from build123d import *

# Parameters (mm, degrees)
F1_DEPTH = 70
F2_R     = 14.3018330781
F3_DEPTH = 87.7
F4_W     = 40
F4_H     = 30
F5_DEPTH = 60
F7_R     = 5
F8_DEPTH = 86.3


with BuildPart() as f1:
    # F0 (on Right) → F1 (new body, symmetric)
    with BuildSketch(Plane.YZ):
        Polygon((0, 30), (0, 0), (-60, 0), (-60, -30), (10, -30), (10, 30), align=None)
    extrude(amount=F1_DEPTH, both=True)

    # F2 (on Right) → F3 (cut, symmetric)
    with BuildSketch(Plane.YZ):
        with Locations((-25, -30)):
            Circle(F2_R)
    extrude(amount=F3_DEPTH, both=True, mode=Mode.SUBTRACT)

    # F4 (on Front) → F5 (join)
    with BuildSketch(Plane.XZ):
        with Locations((20, 15)):
            Rectangle(F4_W, F4_H)
    extrude(amount=F5_DEPTH)

    # F6: F1 across plane


with BuildPart() as f1_1:
    add(f1.part)
    add(f1.part.mirror(Plane.YZ))

    # F7 (on face) → F8 (cut)
    with BuildSketch(Plane.XZ):
        with Locations((-55, 15)):
            Circle(F7_R)
    extrude(amount=-F8_DEPTH, mode=Mode.SUBTRACT)


solid = f1_1.part
Work out the finished part from the listing and answer in its coordinate system (mm). A direction names the side the tool comes from. Round coordinates to 2 decimals unless told otherwise and drop trailing zeros. Order: outer loops, then holes, each group sorted by start corner. A loop starts at its lowest first (then second) coordinate and runs counter-clockwise, first axis right, second up. Notation, with made-up numbers: M 82.5,27 L 102.5,27 A23 ccw 102.5,48 Z; hole C 50.25,-26 d4. An arc over 180 degrees is marked long. Put each result on its own line as item: value. Start each with the question number.
Q1. Section B-B, the plane x = -55 is taken. Write down the section's boundary in (y, z).
Q2. Flat-ended cylindrical pins translate along their axes: pin 1 (2 mm diameter, centred on x = -43, y = -4, fed in from +Z); pin 2 (9 mm diameter, centred on x = 51, z = 14, fed in from -Y); pin 3 (9 mm diameter, centred on y = -22.5, z = 17.5, fed in from +X); pin 4 (8 mm diameter, centred on x = -55, z = 15, fed in from -Y). Find the tip coordinate at first contact, or state that the pin passes through.
Q3. For a pull along X with two mould halves and no side action, classify faces 4 (the flat face through (40, -30, 15)), 5 (the flat face through (-70, -18, -13)), 6 (the cylindrical face through (-59, 5, 12)), 7 (the flat face through (1, 0, -30)) as pulls with the +X half, pulls with the -X half, needs draft (parallel to the pull), parting line crosses it, or undercut.
Q4. Section D-D, the plane y = -25 is taken. Write down the section's boundary in (x, z), and give its area (3 significant figures).
Q5. A tool of negligible diameter and unlimited length cuts with its end or side. For faces 1 (the flat face through (-40, -30, 15)), 2 (the flat face through (1, -50, -30)), 3 (the flat face through (55, -30, 0)), from which of +Z, -Z, +X, -X, +Y, -Y can it reach the whole face along a straight path? Write none if from no direction.
Q6. Section A-A, the plane z = 15 is taken. Write down the section's boundary in (x, y), and give its area (3 significant figures).
Q7. Section C-C, the plane z = 5 is taken. Write down the section's boundary in (x, y), and give its area (3 significant figures).
Q8. Straight lines are drawn through the part: L1, parallel to Z at x = -55, y = 4; L2, parallel to Y at x = 41.5, z = 20.5; L3, parallel to Y at x = -1, z = -19.5. For each, find the intervals that lie inside material, in ascending order. Write a range as [from, to].
Findings below:
1. outline: M -60,-30 L -39.3,-30 A14.3 cw -10.7,-30 L 10,-30 L 10,10 L 0,10 L 0,0 L -60,0 Z; M 0,20 L 10,20 L 10,30 L 0,30 Z
2. pin 1: stops at z = 0
2. pin 2: stops at y = 0
2. pin 3: stops at x = 40
2. pin 4: passes through
3. face 4: pulls with the +X half
3. face 5: pulls with the -X half
3. face 6: undercut
3. face 7: needs draft
4. outline: M -70,-15.7 L 70,-15.7 L 70,0 L 40,0 L 40,30 L -40,30 L -40,0 L -70,0 Z
4. area: 4,600 mm^2
5. face 1: +Z, -X, -Y
5. face 2: -Z, +X, -X, +Y, -Y
5. face 3: +Z, +X, -Y
6. outline: M -70,0 L -60,0 L -60,10 L -70,10 Z; M -50,0 L -40,0 L -40,-60 L 40,-60 L 40,0 L 70,0 L 70,10 L -50,10 Z
6. area: 6,100 mm^2
7. outline: M -70,0 L -40,0 L -40,-60 L 40,-60 L 40,0 L 70,0 L 70,10 L -70,10 Z
7. area: 6,200 mm^2
8. L1: z = [-30, 10], [20, 30]
8. L2: y = [0, 10]
8. L3: y = [-60, -34.71], [-15.29, 10]
